Part model, mm, in its own coordinate system. Round coordinates to 2 decimals unless told otherwise and drop trailing zeros. Write each loop counter-clockwise with the first axis right and the second up, starting at its lowest first coordinate (ties: lowest second). Pieces come first, ordered by that corner, then holes. Notation, with made-up numbers: M 11,20 L 39,20 A16 cw 39,27 Z; hole C 87.5,61.5 d9. An arc over 180 degrees is marked long. Use one line per item in the form item = value. Start each with the question number.
Item 1: Cut at A-A, the plane z = 1.3. Give the cut face in (x, y), then the cut area to 3 significant figures.
Item 2: Probe L1, parallel to Y at x = 86, z = 0.9; L2, parallel to X at y = -2.5, z = 1.5; L3, parallel to Y at x = 304.5, z = 2.7. List the from-to ranges inside material, lowest first.
Item 3: Flat gauge pin, fed straight in: pin 1 Ø2.5 at (x, y) = (-190, 0) entering from -Z. Where does the tip first touch, or does it go through?
from build123d import *

# Parameters (mm, degrees)
F0_W     = 500
F0_H     = 30
F0_R     = 2.05
F0_W_2   = 150
F1_DEPTH = 3


with BuildPart() as f1:
    # F0 (on Top) → F1 (new body)
    with BuildSketch(Plane.XY):
        Rectangle(F0_W, F0_H)
        with BuildLine():
            ThreePointArc((-224.5, 3.5), (-221, 0), (-224.5, -3.5))
            Line((-224.5, -3.5), (-235.5, -3.5))
            ThreePointArc((-235.5, -3.5), (-239, 0), (-235.5, 3.5))
            Line((-235.5, 3.5), (-224.5, 3.5))
        make_face(mode=Mode.SUBTRACT)
        with Locations((-210, 0)):
            Circle(F0_R, mode=Mode.SUBTRACT)
        with Locations((-190, 0)):
            Circle(F0_R, mode=Mode.SUBTRACT)
        with Locations((-134, 0)):
            Circle(F0_R, mode=Mode.SUBTRACT)
        with Locations((86, 0)):
            Circle(F0_R, mode=Mode.SUBTRACT)
        with Locations((325, 0)):
            Rectangle(F0_W_2, F0_H)
        with Locations((306, 0)):
            Circle(F0_R, mode=Mode.SUBTRACT)
        with BuildLine():
            ThreePointArc((385.5, 3.5), (389, 0), (385.5, -3.5))
            Line((385.5, -3.5), (374.5, -3.5))
            ThreePointArc((374.5, -3.5), (371, 0), (374.5, 3.5))
            Line((374.5, 3.5), (385.5, 3.5))
        make_face(mode=Mode.SUBTRACT)
    extrude(amount=F1_DEPTH)


solid = f1.part
Model answer:
q1.outline = M -250,-15 L 400,-15 L 400,15 L -250,15 Z; hole M -235.5,-3.5 L -224.5,-3.5 A3.5 ccw -224.5,3.5 L -235.5,3.5 A3.5 ccw Z; hole C -210,0 d4.1; hole C -190,0 d4.1; hole C -134,0 d4.1; hole C 86,0 d4.1; hole C 306,0 d4.1; hole M 374.5,-3.5 L 385.5,-3.5 A3.5 ccw 385.5,3.5 L 374.5,3.5 A3.5 ccw Z
q1.area = 19,200 mm²
q2.L1 = -15 to -2.05, 2.05 to 15
q2.L2 = -250 to -237.95, -222.05 to 372.05, 387.95 to 400
q2.L3 = -15 to -1.4, 1.4 to 15
q3.pin_1 = through
